from build123d import *

# Parameters (mm, degrees)
BOSS_EXTRUDE1_DEPTH = 10
SKETCH2_R           = 38
BOSS_EXTRUDE2_DEPTH = 41
CUT_EXTRUDE1_START  = 10
SKETCH3_W           = 76
SKETCH3_H           = 5
CUT_EXTRUDE1_DEPTH  = 50
CUT_EXTRUDE2_START  = -10
SKETCH4_W           = 76
SKETCH4_H           = 5
CUT_EXTRUDE2_DEPTH  = 41


with BuildPart() as part:
    # Sketch1 → Boss-Extrude1 (new body)
    with BuildSketch(Plane(origin=(0, 0, 0), x_dir=(1, 0, 0), z_dir=(0, 1, 0))):
        Polygon((-100, 150), (-150, 85), (-150, -85), (-100, -150), (100, -150), (150, -85), (150, 85), (100, 150), align=None)
    extrude(amount=BOSS_EXTRUDE1_DEPTH)

    # Sketch2 → Boss-Extrude2 (add)
    with BuildSketch(Plane(origin=(0, 10, 0), x_dir=(1, 0, 0), z_dir=(0, 1, 0))):
        with Locations(Location((0, 0, 0), (0, 0, 270))):
            Circle(SKETCH2_R)
    extrude(amount=BOSS_EXTRUDE2_DEPTH)

    # Sketch3 → Cut-Extrude1 (cut)
    with BuildSketch(Plane.XY.offset(CUT_EXTRUDE1_START)):
        with Locations((0, 33.5)):
            Rectangle(SKETCH3_W, SKETCH3_H)
    extrude(amount=CUT_EXTRUDE1_DEPTH, mode=Mode.SUBTRACT)

    # Sketch4 → Cut-Extrude2 (cut)
    with BuildSketch(Plane.XY.offset(CUT_EXTRUDE2_START)):
        with Locations((0, 33.5)):
            Rectangle(SKETCH4_W, SKETCH4_H)
    extrude(amount=-CUT_EXTRUDE2_DEPTH, mode=Mode.SUBTRACT)


solid = part.part
Model file for the job. Use its own axes, mm. A direction names the side the tool comes from. Give positions to 0.01 mm unless a question says otherwise; leave off trailing zeros. Write each loop counter-clockwise with the first axis right and the second up, starting at its lowest first coordinate (ties: lowest second). Pieces come first, ordered by that corner, then holes. Notation, with made-up numbers: M -5,-1.5 L 30,-1.5 A14 cw 30,7.5 Z; hole C 63.5,53 d3. An arc over 180 degrees is marked long. One line per item, written item: value. Start each with the question number.
Q1. Saw through at B-B, the plane x = 0. Write the cut outline in (y, z), plus the area to 3 significant figures.
Q2. Saw through at A-A, the plane z = -29. Write the cut outline in (x, y), plus the area to 3 significant figures.
Q3. 3-axis set-ups, long thin cutter, end or side, ignore diameter. For faces 1 (the flat face through (-124.65, 4.93, -117.955)), 2 (the flat face through (31, 10, -35)), 3 (the flat face through (-1, 5, 150)), 4 (the flat face through (-1, 36, 21)), 5 (the flat face through (-1, 36, -21)): which of +Z, -Z, +X, -X, +Y, -Y reach the whole face in a straight line?
Q4. Probe probe 1 along Y at (x, z) = (-19.5, -54); probe 2 along Z at (x, y) = (13.5, 32); probe 3 along X at (y, z) = (40.5, -14.5). List the from-to ranges inside material, lowest first. Write a range as [from, to].
Q5. Saw through at D-D, the plane z = -63. Write the cut outline in (x, y).
Q6. Saw through at C-C, the plane y = 25. Write the cut outline in (x, z), plus the area to 3 significant figures.
Q7. Drop flat-ended pins along their axis: pin 1 Ø2.5 at (x, y) = (4.5, 32.5) entering from +Z; pin 2 Ø2 at (x, z) = (3, 20.5) entering from -Y; pin 3 Ø5 at (y, z) = (38, 17.5) entering from +X; pin 4 Ø4 at (x, z) = (33.5, -58.5) entering from +Y. Give the stop position or say it passes through.
Q8. Two-plate mould, pull along Y, no slides. Class faces 6 (the flat face through (125.35, 4.93, -117.045)), 7 (the flat face through (1, 51, -1)), 8 (the flat face through (-1, 31, -21)): +Y half, -Y half, draft (parallel to the pull), parting line (faces both ways), or undercut.
Output values:
1. outline: M 0,-150 L 10,-150 L 10,-38 L 31,-38 L 31,-10 L 36,-10 L 36,-38 L 51,-38 L 51,38 L 36,38 L 36,10 L 31,10 L 31,38 L 10,38 L 10,150 L 0,150 Z
1. area: 5,840 mm²
2. outline: M -150,0 L 150,0 L 150,10 L 24.56,10 L 24.56,31 L -24.56,31 L -24.56,10 L -150,10 Z; M -24.56,36 L 24.56,36 L 24.56,51 L -24.56,51 Z
2. area: 4,770 mm²
3. face 1: -Z, -X, +Y, -Y
3. face 2: +Y
3. face 3: +Z, +X, -X, +Y, -Y
3. face 4: +Z, +X, -X
3. face 5: -Z, +X, -X
4. probe 1: y = [0, 10]
4. probe 2: z = [-10, 10]
4. probe 3: x = [-35.12, 35.12]
5. outline: M -150,0 L 150,0 L 150,10 L -150,10 Z
6. outline: C 0,0 d76
6. area: 4,540 mm²
7. pin 1: stops at z = 10
7. pin 2: stops at y = 0
7. pin 3: stops at x = 34.91
7. pin 4: stops at y = 10
8. face 6: draft
8. face 7: +Y half
8. face 8: undercut
